Verification items for the finished model (mm, model axes). A direction names the side the tool comes from. Give positions to 0.01 mm unless a question says otherwise; leave off trailing zeros. Write each loop counter-clockwise with the first axis right and the second up, starting at its lowest first coordinate (ties: lowest second). Pieces come first, ordered by that corner, then holes.
from build123d import *

# Parameters (mm, degrees)
CROQUIS1_R                 = 25
SALIENTE_EXTRUIR1_DEPTH    = 3
CROQUIS2_R                 = 10
SALIENTE_EXTRUIR2_DEPTH    = 10
CROQUIS3_R                 = 4
CORTAR_EXTRUIR1_DEPTH      = 38.669616404
CROQUIS4_R                 = 2
CORTAR_EXTRUIR2_DEPTH      = 37.742346142
CORTAR_EXTRUIR3_DEPTH      = 38.669616404
CORTAR_EXTRUIR3_DEPTH_BACK = 38.669616404
CROQUIS5_R                 = 2


with BuildPart() as part:
    # Croquis1 → Saliente-Extruir1 (new body)
    with BuildSketch(Plane.XY):
        Circle(CROQUIS1_R)
    extrude(amount=SALIENTE_EXTRUIR1_DEPTH)

    # Croquis2 → Saliente-Extruir2 (add)
    with BuildSketch(Plane.XY.offset(3)):
        Circle(CROQUIS2_R)
    extrude(amount=SALIENTE_EXTRUIR2_DEPTH)

    # Croquis3 → Cortar-Extruir1 (cut, through all)
    with BuildSketch(Plane.XY.offset(13)):
        Circle(CROQUIS3_R)
    extrude(amount=-CORTAR_EXTRUIR1_DEPTH, mode=Mode.SUBTRACT)

    # Croquis4 → Cortar-Extruir2 (cut, through all)
    with BuildSketch(Plane.XY.offset(3)):
        with Locations((-4.65167861, 15.308882589)):
            Circle(CROQUIS4_R)
        with Locations((15.308882589, 4.65167861)):
            Circle(CROQUIS4_R)
        with Locations((4.65167861, -15.308882589)):
            Circle(CROQUIS4_R)
        with Locations((-15.308882589, -4.65167861)):
            Circle(CROQUIS4_R)
    extrude(amount=-CORTAR_EXTRUIR2_DEPTH, mode=Mode.SUBTRACT)

    # Croquis5 → Cortar-Extruir3 (cut, two sides: drawn at the far end of the back side and taken through both)
    with BuildSketch(Plane(origin=(0, 0, 0), x_dir=(0, 0, -1), z_dir=(1, 0, 0)).offset(-CORTAR_EXTRUIR3_DEPTH_BACK)):
        with Locations((-8, 0)):
            Circle(CROQUIS5_R)
    extrude(amount=CORTAR_EXTRUIR3_DEPTH + CORTAR_EXTRUIR3_DEPTH_BACK, mode=Mode.SUBTRACT)


solid = part.part
Item 1: Sectioned sample at C-C on z = 8. Record the cut outline in (x, y), then the cut area to 3 significant figures.
Answer key:
outline: (-9.8, -2) arc R10 ccw to (9.8, -2) - (3.46, -2) arc R4 cw to (-3.46, -2) - close; (-9.8, 2) - (-3.46, 2) arc R4 cw to (3.46, 2) - (9.8, 2) arc R10 ccw to start
area: 215 mm2
Item 2: Sectioned sample at D-D on y = 6. Record the cut outline in (x, z).
Answer key:
outline: (-24.27, 0) - (13.83, 0) - (13.83, 3) - (8, 3) - (8, 13) - (-8, 13) - (-8, 3) - (-24.27, 3) - close; (16.79, 0) - (24.27, 0) - (24.27, 3) - (16.79, 3) - close
Item 3: Scan lines: line 1 along Z through (x, y) = (8, 0); line 2 along X through (y, z) = (3.5, 2.5); line 3 along Y through (x, z) = (-0.5, 7.25). Record each from-to range of solid material in increasing order.
Answer key:
line 1: z = 0 to 6, 10 to 13
line 2: x = -24.75 to -1.94, 1.94 to 13.67, 16.94 to 24.75
line 3: y = -9.99 to -3.97, 3.97 to 9.99
Item 4: Sectioned sample at B-B on x = 0. Record the cut outline in (y, z).
Answer key:
outline: (-25, 0) - (-4, 0) - (-4, 13) - (-10, 13) - (-10, 3) - (-25, 3) - close; (4, 0) - (25, 0) - (25, 3) - (10, 3) - (10, 13) - (4, 13) - close
Item 5: Depth check by flat-ended pin: pin 1 (2 mm diameter, centred on y = 5.5, z = 2.5, fed in from -X); pin 2 (1.5 mm diameter, centred on x = 1.5, z = 1.5, fed in from -Y); pin 3 (5 mm diameter, centred on y = 15.5, z = 2.5, fed in from +X). Enter the tip coordinate at first touch or a pass-through.
Answer key:
pin 1: stops at x = -24.59
pin 2: stops at y = -24.99
pin 3: stops at x = 21.35
Item 6: Sectioned sample at A-A on y = 0. Record the cut outline in (x, z), then the cut area to 3 significant figures.
Answer key:
outline: (-25, 0) - (-4, 0) - (-4, 6) - (-10, 6) - (-10, 3) - (-25, 3) - close; (-10, 10) - (-4, 10) - (-4, 13) - (-10, 13) - close; (4, 0) - (25, 0) - (25, 3) - (10, 3) - (10, 6) - (4, 6) - close; (4, 10) - (10, 10) - (10, 13) - (4, 13) - close
area: 198 mm2
Item 7: Set-up check for faces 5 (the face through (-14.39, -6.43, 1.52)), 6 (the face through (11, 0, 3)): record each of +Z, -Z, +X, -X, +Y, -Y from which the full face is reachable in a straight line by a thin tool's end or side.
Answer key:
face 5: +Z, -Z
face 6: +Z
Item 8: Release check for a two-part mould opening along Y. For faces 1 (the face through (3.178, -13.957, 1.521)), 2 (the face through (-0.1, -4.3, 13)), 3 (the face through (23.846, 7.509, 1.479)), 4 (the face through (13.31, 4.74, 1.52)) record: released by +Y, released by -Y, zero draft, split by the parting line, or undercut.
Answer key:
face 1: undercut
face 2: zero draft
face 3: split by the parting line
face 4: undercut
